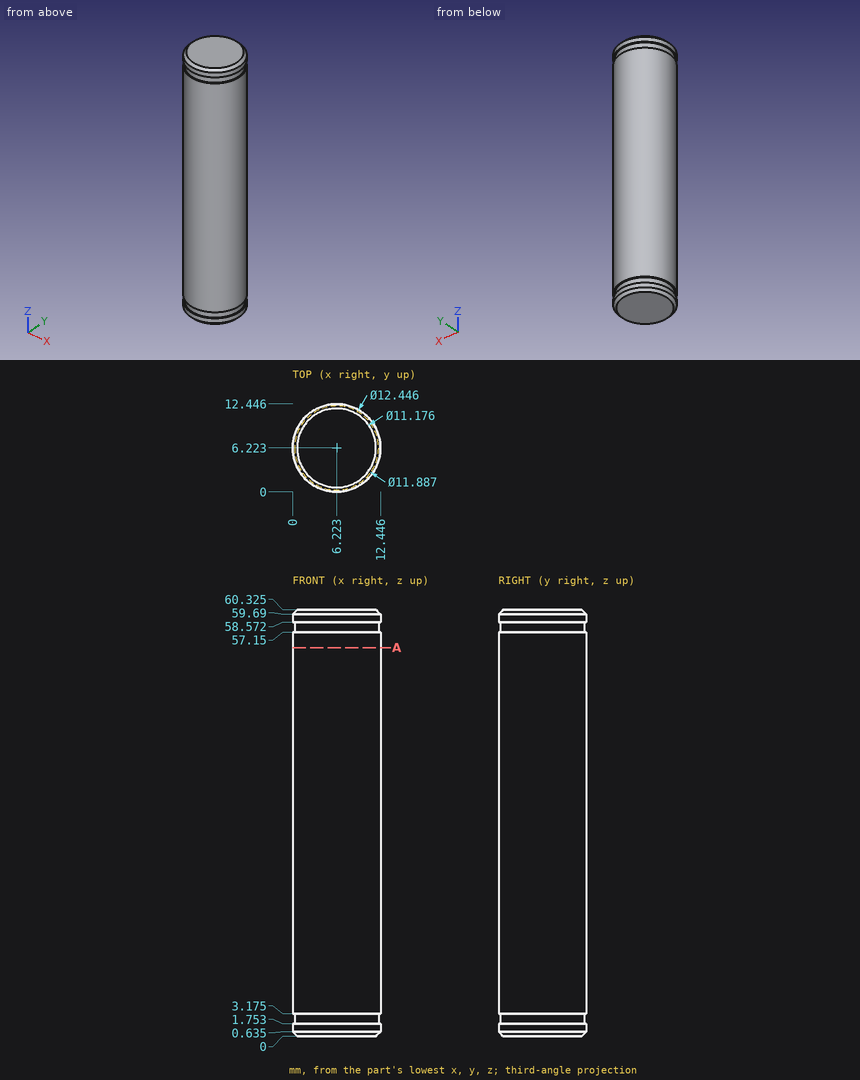
Source: three-view drawing plus pictorial views. Frame: mm from the lowest corner of the part. Round coordinates to 2 decimals unless told otherwise and drop trailing zeros. Loops run counter-clockwise (first coordinate to the right, second up) from the corner with the lowest first, then second, coordinate; pieces in that order, holes last.
Q1. Ray query, line 1 (Y direction, x = 6, z = 41.5); line 2 (X direction, y = 7.25, z = 53) (1 decimal); line 3 (X direction, y = 11.25, z = 18) (1 decimal). Return the intervals inside material, ascending.
Q2. Section A-A, the plane z = 55. Return loops of the section in (x, y).
Q3. First-contact query: P1, Ø6, axis at y = 7.5, z = 44, coming from the -X side; P2, Ø6, axis at x = 10.5, z = 26, coming from the +Y side; P3, Ø4, axis at x = 2, z = 22, coming from the +Y side (1 decimal). Flat tips, straight axial feed; report the tip coordinate or a pass-through.
Solutions:
1. line 1: y = 0 to 12.44
1. line 2: x = 0.1 to 12.4
1. line 3: x = 2.6 to 9.9
2. outline: circle Ø12.45 at (6.22, 6.22)
3. P1: stops at x = 0
3. P2: stops at y = 12.31
3. P3: stops at y = 12
